Autodesk Inventor part; units mm, degrees
ref_plane "YZ Plane" through (0, 0, 0) normal (1, 0, 0) x (0, 1, 0)
ref_plane "XZ Plane" through (0, 0, 0) normal (0, 1, 0) x (-1, 0, 0)
ref_plane "XY Plane" through (0, 0, 0) normal (0, 0, 1) x (1, 0, 0)
sketch "スケッチ1" plane through (0, 0, 0) normal (1, 0, 0) x (0, 1, 0)
  line L0 (0, 0) -> (-61.5, 0)
  line L1 (-61.5, 0) -> (-61.5, -116)
  line L2 (-61.5, -116) -> (0, -116)
  line L3 (0, -116) -> (0, 0)
  dimension "d0" = 61.5
  dimension "d1" = 116
extrude "押し出し1" add sketch "スケッチ1" along normal blind 5.5
sketch "スケッチ2" plane through (0, 0, 0) normal (-1, 0, 0) x (0, 0, 1)
  line L0 (-116, -61.5) -> (-116, 0)
  line L1 (-116, 0) -> (0, 0)
  line L2 (0, -61.5) -> (-116, -61.5)
  line L3 (0, 0) -> (0, -61.5)
  point P0 (-108.5, -7.5)
  point P1 (-7.5, -7.5)
  point P2 (-7.5, -54)
  point P3 (-108.5, -54)
  dimension "d4" = 7.5
  dimension "d5" = 7.5
  dimension "d6" = 7.5
  dimension "d7" = 7.5
  dimension "d8" = 7.5
  dimension "d9" = 7.5
  dimension "d10" = 7.5
  dimension "d11" = 7.5
hole "穴1" at (0, -7.5, -108.5) at (0, -7.5, -7.5) at (0, -54, -7.5) at (0, -54, -108.5) direction (1, 0, 0) diameter 3 end through all
fillet "フィレット1" radius 7.5 4 edges at (2.75, 0, 0) (2.75, -61.5, 0) (2.75, -61.5, -116) (2.75, 0, -116)
sketch "スケッチ3" plane through (0, 0, 0) normal (-1, 0, 0) x (0, 0, 1)
  line L0 (0, -7.5) -> (0, -54)
  line L1 (-116, -54) -> (-116, -7.5)
  line L2 (-108.5, 0) -> (-7.5, 0)
  point P0 (0, 0)
  point P1 (-58, -14.5)
  point P2 (-58, 65.5)
  dimension "d20" = 116
  dimension "d21" = 58
  dimension "d49" = 65.5
  dimension "d50" = 80
hole "穴2" at (0, -14.5, -58) direction (1, 0, 0) diameter 12 end through all
sketch "スケッチ4" plane through (0, 0, 0) normal (-1, 0, 0) x (0, 0, 1)
  circle A0 centre (-58, -21.5) radius 15.5
  line L0 (-58, -21.5) -> (-42.5, -21.5)
  line L1 (-58, -21.5) -> (-65.75, -34.9234)
  line L2 (-58, -21.5) -> (-42.5, -21.5) construction
  line L3 (-58, -21.5) -> (-65.75, -8.0766)
  circle A1 centre (-58, -14.5) radius 6
  point P0 (0, 0)
  dimension "d31" = 31
  dimension "d32" = 120
  dimension "d33" = 120
  dimension "d51" = 7
  dimension "d52" = 0
hole "穴3" at (0, -21.5, -42.5) at (0, -34.9234, -65.75) at (0, -8.0766, -65.75) direction (1, 0, 0) diameter 3 end through all
sketch "スケッチ5" plane through (0, 0, 0) normal (-1, 0, 0) x (0, 0, 1)
  circle A0 centre (-58, -14.5) radius 6
  circle A1 centre (-58, 65.5) radius 70
  point P0 (0, 0)
  dimension "d42" = 65.5
  dimension "d43" = 58
  dimension "d44" = 58
  dimension "d45" = 140
extrude "押し出し2" cut sketch "スケッチ5" against normal through all contours A1
fillet "フィレット2" radius 15 2 edges at (2.75, 0, -33.3069) (2.75, 0, -82.6931)
sketch "スケッチ6" plane through (0, 0, 0) normal (-1, 0, 0) x (0, 0, 1)
  circle A0 centre (-7.5, -7.5) radius 1.5
  line L0 (-30.7099, 0) -> (-7.5, 0)
  line L1 (0, -7.5) -> (0, -54)
  point P0 (0, 0)
  point P1 (-15.5, -7.5)
  point P2 (-20.5, -7.5)
  point P3 (-25.5, -7.5)
  point P4 (-15.5, -12.5)
  point P5 (-20.5, -12.5)
  point P6 (-25.5, -12.5)
  point P7 (-15.5, -17.5)
  point P8 (-20.5, -17.5)
  point P9 (-25.5, -17.5)
  point P10 (-15.5, -22.5)
  point P11 (-20.5, -22.5)
  point P12 (-25.5, -22.5)
  point P13 (-15.5, -27.5)
  point P14 (-20.5, -27.5)
  point P15 (-25.5, -27.5)
  point P16 (-15.5, -32.5)
  point P17 (-20.5, -32.5)
  point P18 (-25.5, -32.5)
  point P19 (-15.5, -37.5)
  point P20 (-20.5, -37.5)
  point P21 (-25.5, -37.5)
  point P22 (-15.5, -42.5)
  point P23 (-20.5, -42.5)
  point P24 (-25.5, -42.5)
  point P25 (-15.5, -47.5)
  point P26 (-20.5, -47.5)
  point P27 (-25.5, -47.5)
  point P28 (-15.5, -52.5)
  point P29 (-20.5, -52.5)
  point P30 (-25.5, -52.5)
  point P31 (-30.5, -7.5)
  point P32 (-30.5, -12.5)
  point P33 (-30.5, -17.5)
  point P34 (-30.5, -22.5)
  point P35 (-30.5, -27.5)
  point P36 (-30.5, -32.5)
  point P37 (-30.5, -37.5)
  point P38 (-30.5, -42.5)
  point P39 (-30.5, -47.5)
  point P40 (-30.5, -52.5)
  dimension "d53" = 8
  dimension "d54" = 7.5
  dimension "d64" = 5
  dimension "d69" = 15.5
  dimension "d72" = 5
  dimension "d79" = 5
hole "穴4" at (0, -7.5, -15.5) at (0, -7.5, -20.5) at (0, -7.5, -25.5) at (0, -12.5, -15.5) at (0, -12.5, -20.5) at (0, -12.5, -25.5) at (0, -17.5, -15.5) at (0, -17.5, -20.5) at (0, -17.5, -25.5) at (0, -22.5, -15.5) at (0, -22.5, -20.5) at (0, -22.5, -25.5) at (0, -27.5, -15.5) at (0, -27.5, -20.5) at (0, -27.5, -25.5) at (0, -32.5, -15.5) at (0, -32.5, -20.5) at (0, -32.5, -25.5) at (0, -37.5, -15.5) at (0, -37.5, -20.5) at (0, -37.5, -25.5) at (0, -42.5, -15.5) at (0, -42.5, -20.5) at (0, -42.5, -25.5) at (0, -47.5, -15.5) at (0, -47.5, -20.5) at (0, -47.5, -25.5) at (0, -52.5, -15.5) at (0, -52.5, -20.5) at (0, -52.5, -25.5) at (0, -7.5, -30.5) at (0, -12.5, -30.5) at (0, -17.5, -30.5) at (0, -22.5, -30.5) at (0, -27.5, -30.5) at (0, -32.5, -30.5) at (0, -37.5, -30.5) at (0, -42.5, -30.5) at (0, -47.5, -30.5) at (0, -52.5, -30.5) direction (1, 0, 0) diameter 3 end through all
sketch "スケッチ7" plane through (0, 0, 0) normal (-1, 0, 0) x (0, 0, 1)
  circle A0 centre (-87.9685, -8.6747) radius 4
  circle A1 centre (-58, 65.5) radius 80
  line L0 (0, -7.5) -> (0, -54)
  line L1 (-116, -54) -> (-116, -7.5)
  circle A2 centre (-58, -14.5) radius 6
  line L2 (-58, 65.5) -> (-87.9685, -8.6747)
  line L3 (-58, 65.5) -> (-58, -14.5)
  point P0 (0, 0)
  dimension "d94" = 160
  dimension "d91" = 8
  dimension "d95" = 116
  dimension "d96" = 58
  dimension "d97" = 80
  dimension "d98" = 22
extrude "押し出し3" cut sketch "スケッチ7" against normal through all contours A0 A1 L2 | L2 A1 A0 | A0 A1
equation "\"d96\" = 0.5 * d95"
equation "\"d97\" = 0.5 * d94"
properties part number "ロボットベースT5.5" material "木材 (クルミ材)"
Geometry check sheet. Reference: the model listing, model coordinates, mm. A direction names the side the tool comes from. Give positions to 0.01 mm unless a question says otherwise; leave off trailing zeros. Write each loop counter-clockwise with the first axis right and the second up, starting at its lowest first coordinate (ties: lowest second). Pieces come first, ordered by that corner, then holes.
1) Release check for a two-part mould opening along Z. For faces 3 (the cylindrical face through (2.79, -23.51, -21.61)), 4 (the cylindrical face through (2.788, -59.245, -2.139)) record: pulls with the +Z half, pulls with the -Z half, needs draft (parallel to the pull), parting line crosses it, or undercut.
2) Material ranges on L1, parallel to Z at x = 1.4, y = -42.5; L2, parallel to Y at x = 1.6, z = -7.5; L3, parallel to Z at x = 3.65, y = -54.5, recorded low to high.
3) Section check C-C, the plane z = -42.5. Record the boundary of the cut face in (x, y).
4) Section check A-A, the plane y = -47.5. Record the boundary of the cut face in (x, z), and give its area (3 significant figures).
5) Section check B-B, the plane z = -15.5. State how many separate pieces and enclosed holes the cut face has, and give its area (3 significant figures).
6) Access from +Z, -Z, +X, -X, +Y, -Y to the whole of each face (thin tool, end or side, straight path). Record for faces 1 (the cylindrical face through (2.8, -36.6, -16.7)), 2 (the cylindrical face through (2.712, -0.205, -82.816)).
Computed:
1. face 3: undercut
1. face 4: pulls with the +Z half
2. L1: z = -116 to -32, -29 to -27, -24 to -22, -19 to -17, -14 to 0
2. L2: y = -61.5 to -55.5, -52.5 to -9, -6 to 0
2. L3: z = -115.98 to -109.91, -107.09 to -8.91, -6.09 to -0.02
3. outline: (0, -61.5) - (5.5, -61.5) - (5.5, -23) - (0, -23) - close; (0, -20) - (5.5, -20) - (5.5, -2.76) - (0, -2.76) - close
4. outline: (0, -116) - (5.5, -116) - (5.5, -32) - (0, -32) - close; (0, -29) - (5.5, -29) - (5.5, -27) - (0, -27) - close; (0, -24) - (5.5, -24) - (5.5, -22) - (0, -22) - close; (0, -19) - (5.5, -19) - (5.5, -17) - (0, -17) - close; (0, -14) - (5.5, -14) - (5.5, 0) - (0, 0) - close
4. area: 572 mm2
5. separate pieces: 11
5. enclosed holes: 0
5. area: 173 mm2
6. face 1: +X, -X
6. face 2: +X, -X, +Y
